The listing builds one solid part. Answer for the finished solid, in the listing's coordinates (mm). A direction names the side the tool comes from. Coordinates: 2 decimals unless noted, no trailing zeros. Write each loop counter-clockwise with the first axis right and the second up, starting at its lowest first coordinate (ties: lowest second). Pieces come first, ordered by that corner, then holes.
from build123d import *

# Parameters (mm, degrees)
F1_DEPTH = 25.4
F2_R     = 6.35
F3_DEPTH = 12.701
F5_DEPTH = 50.801
F7_DEPTH = 12.701


with BuildPart() as f1:
    # F0 (on Front) → F1 (new body)
    with BuildSketch(Plane.XZ):
        Polygon((-70.5749627616, 18.429359109), (-70.5749627616, 5.729359109), (5.6250372384, 5.729359109), (5.6250372384, 18.429359109), (-19.7749627616, 18.429359109), (-19.7749627616, 50.179359109), (-45.1749627616, 50.179359109), (-45.1749627616, 18.429359109), align=None)
    extrude(amount=F1_DEPTH)

    # F2 (on face) → F3 (cut, through all)
    with BuildSketch(Plane.XY.offset(18.429359109)):
        with Locations((-7.0749627616, -12.7)):
            Circle(F2_R)
        with BuildLine():
            ThreePointArc((5.6250372384, -12.7), (1.9052933594, -21.6802561211), (-7.0749627616, -25.4))
            Line((-7.0749627616, -25.4), (5.6250372384, -25.4))
            Line((5.6250372384, -25.4), (5.6250372384, -12.7))
        make_face()
        with BuildLine():
            ThreePointArc((-7.0749627616, 0), (1.9052933594, -3.7197438789), (5.6250372384, -12.7))
            Line((5.6250372384, -12.7), (5.6250372384, 0))
            Line((5.6250372384, 0), (-7.0749627616, 0))
        make_face()
    extrude(amount=-F3_DEPTH, mode=Mode.SUBTRACT)

    # F4 (on face) → F5 (cut, through all)
    with BuildSketch(Plane.YZ.offset(-19.7749627616)):
        with BuildLine():
            ThreePointArc((-19.05, 37.479359109), (-12.7, 31.129359109), (-6.35, 37.479359109))
            ThreePointArc((-6.35, 37.479359109), (-8.2098719395, 41.9694871695), (-12.7, 43.829359109))
            ThreePointArc((-12.7, 43.829359109), (-17.1901280605, 41.9694871695), (-19.05, 37.479359109))
        make_face()
        with BuildLine():
            ThreePointArc((-25.4, 37.479359109), (-21.6802561211, 46.45961523), (-12.7, 50.179359109))
            Line((-12.7, 50.179359109), (-25.4, 50.179359109))
            Line((-25.4, 50.179359109), (-25.4, 37.479359109))
        make_face()
        with BuildLine():
            ThreePointArc((-12.7, 50.179359109), (-3.7197438789, 46.45961523), (0, 37.479359109))
            Line((0, 37.479359109), (0, 50.179359109))
            Line((0, 50.179359109), (-12.7, 50.179359109))
        make_face()
    extrude(amount=-F5_DEPTH, mode=Mode.SUBTRACT)

    # F6 (on face) → F7 (cut, through all)
    with BuildSketch(Plane.XY.offset(18.429359109)):
        with BuildLine():
            ThreePointArc((-70.5749627616, -12.60582854), (-66.8220875421, -3.6863877476), (-57.8749627616, 0))
            Line((-57.8749627616, 0), (-70.5749627616, 0))
            Line((-70.5749627616, 0), (-70.5749627616, -12.60582854))
        make_face()
        with BuildLine():
            Line((-70.5749627616, -25.4), (-57.8749627616, -25.4))
            ThreePointArc((-57.8749627616, -25.4), (-66.8220875421, -21.7136122524), (-70.5749627616, -12.79417146))
            Line((-70.5749627616, -12.79417146), (-70.5749627616, -25.4))
        make_face()
        with BuildLine():
            ThreePointArc((-57.8749627616, -19.05), (-53.3848347011, -17.1901280605), (-51.5249627616, -12.7))
            ThreePointArc((-51.5249627616, -12.7), (-53.3848347011, -8.2098719395), (-57.8749627616, -6.35))
            ThreePointArc((-57.8749627616, -6.35), (-62.3650908222, -8.2098719395), (-64.2249627616, -12.7))
            ThreePointArc((-64.2249627616, -12.7), (-62.3650908222, -17.1901280605), (-57.8749627616, -19.05))
        make_face()
    extrude(amount=-F7_DEPTH, mode=Mode.SUBTRACT)


solid = f1.part
1. Flat-ended cylindrical pins translate along their axes: P1, Ø10, axis at y = -7.5, z = 16, coming from the -X side; P2, Ø4, axis at x = -30, y = -7, coming from the +Z side; P3, Ø1, axis at x = -34.5, y = -21, coming from the +Z side. Find the tip coordinate at first contact, or state that the pin passes through.
Results found:
P1: stops at x = -70.57
P2: stops at z = 49.63
P3: stops at z = 47.5
2. Section C-C on y = -11.5 is taken. Give the vertices of the cut face in (x, z).
Results found:
outline: (-70.52, 5.73) - (-64.11, 5.73) - (-64.11, 18.43) - (-70.52, 18.43) - close; (-51.64, 5.73) - (-13.31, 5.73) - (-13.31, 18.43) - (-19.77, 18.43) - (-19.77, 31.24) - (-45.17, 31.24) - (-45.17, 18.43) - (-51.64, 18.43) - close; (-45.17, 43.71) - (-19.77, 43.71) - (-19.77, 50.12) - (-45.17, 50.12) - close; (-0.84, 5.73) - (5.57, 5.73) - (5.57, 18.43) - (-0.84, 18.43) - close
3. Section A-A on x = -25 is taken. Give the vertices of the cut face in (y, z), then the cut area to 3 significant figures.
Results found:
outline: (-25.4, 5.73) - (0, 5.73) - (0, 37.48) arc R12.7 ccw to (-25.4, 37.48) - close; hole circle Ø12.7 at (-12.7, 37.48)
area: 933 mm2
4. Section B-B on z = 14 is taken. Give the vertices of the cut face in (x, y).
Results found:
outline: (-70.57, -12.79) arc R12.7 ccw to (-57.87, -25.4) - (-7.07, -25.4) arc R12.7 ccw to (-7.07, 0) - (-57.87, 0) arc R12.7 ccw to (-70.57, -12.61) - close; hole circle Ø12.7 at (-57.87, -12.7); hole circle Ø12.7 at (-7.07, -12.7)
5. A tool of negligible diameter and unlimited length cuts with its end or side. For faces 5 (the flat face through (-45.175, -10, 31)), 6 (the flat face through (-15, -13, 18.429)), 7 (the flat face through (-33, -13, 5.729)), from which of +Z, -Z, +X, -X, +Y, -Y can it reach the whole face along a straight path? Write none if from no direction.
Results found:
face 5: +Z, -X, +Y, -Y
face 6: +Z, +X, +Y, -Y
face 7: -Z, +X, -X, +Y, -Y
6. For a pull along X with two mould halves and no side action, classify faces 1 (the flat face through (-52.1, -9.7, 18.429)), 2 (the flat face through (-19.775, -12.5, 30.6)), 3 (the cylindrical face through (-1.21, -15.13, 12.17)), 4 (the cylindrical face through (-66.92, -3.785, 12.168)) as pulls with the +X half, pulls with the -X half, needs draft (parallel to the pull), parting line crosses it, or undercut.
Results found:
face 1: needs draft
face 2: pulls with the +X half
face 3: undercut
face 4: pulls with the -X half
7. Find the intervals of material crossed by L1, parallel to X at y = -11.25, z = 8.5; L2, parallel to X at y = -19.75, z = 41; L3, parallel to Y at x = -54.5, z = 10, in increasing order.
Results found:
L1: x = -70.49 to -64.06, -51.69 to -13.26, -0.89 to 5.54
L2: x = -45.17 to -19.77
L3: y = -25.4 to -18.08, -7.32 to 0
8. Section D-D on x = -54.5 is taken. Give the vertices of the cut face in (y, z), then the cut area to 3 significant figures.
Results found:
outline: (-25.4, 5.73) - (-18.08, 5.73) - (-18.08, 18.43) - (-25.4, 18.43) - close; (-7.32, 5.73) - (0, 5.73) - (0, 18.43) - (-7.32, 18.43) - close
area: 186 mm2
